from build123d import *

# Parameters (mm, degrees)
SKETCH1_W           = 160
SKETCH1_H           = 180
BOSS_EXTRUDE1_DEPTH = 19.05
SKETCH2_W           = 160
SKETCH2_H           = 180
SKETCH2_W_2         = 147.3
SKETCH2_H_2         = 167.3
BOSS_EXTRUDE2_DEPTH = 44.680000048
SKETCH3_R           = 6.253999938
CUT_EXTRUDE1_DEPTH  = 12.7
SKETCH4_W           = 19.05
SKETCH4_H           = 19.05
SKETCH4_R           = 3.175
BOSS_EXTRUDE3_DEPTH = 12.7


with BuildPart() as part:
    # Sketch1 → Boss-Extrude1 (new body)
    with BuildSketch(Plane(origin=(0, 0, 0), x_dir=(1, 0, 0), z_dir=(0, 1, 0))):
        Rectangle(SKETCH1_W, SKETCH1_H)
    extrude(amount=BOSS_EXTRUDE1_DEPTH)

    # Sketch2 → Boss-Extrude2 (add)
    with BuildSketch(Plane(origin=(0, 19.05, 0), x_dir=(1, 0, 0), z_dir=(0, 1, 0))):
        Rectangle(SKETCH2_W, SKETCH2_H)
        Rectangle(SKETCH2_W_2, SKETCH2_H_2, mode=Mode.SUBTRACT)
    extrude(amount=BOSS_EXTRUDE2_DEPTH)

    # Sketch3 → Cut-Extrude1 (cut)
    with BuildSketch(Plane(origin=(0, 19.05, 0), x_dir=(1, 0, 0), z_dir=(0, 1, 0))):
        with Locations(Location((38.41, -45.55, 0), (0, 0, 270))):
            Circle(SKETCH3_R)
        with Locations(Location((23.17, -45.55, 0), (0, 0, 270))):
            Circle(SKETCH3_R)
        with Locations(Location((38.41, -30.31, 0), (0, 0, 270))):
            Circle(SKETCH3_R)
        with Locations(Location((23.17, -30.31, 0), (0, 0, 270))):
            Circle(SKETCH3_R)
    extrude(amount=-CUT_EXTRUDE1_DEPTH, mode=Mode.SUBTRACT)

    # Sketch4 → Boss-Extrude3 (add)
    # profile 1 of 4: a face of its own
    with BuildSketch(Plane.XZ):
        with Locations((-89.525, -50.08)):
            Rectangle(SKETCH4_W, SKETCH4_H)
        with Locations(Location((-89.525, -50.08, 0), (0, 0, 270))):
            Circle(SKETCH4_R, mode=Mode.SUBTRACT)
    # profile 2 of 4: a face of its own
    with BuildSketch(Plane.XZ):
        with Locations((-89.525, 51.52)):
            Rectangle(SKETCH4_W, SKETCH4_H)
        with Locations(Location((-89.525, 51.52, 0), (0, 0, 270))):
            Circle(SKETCH4_R, mode=Mode.SUBTRACT)
    # profile 3 of 4: a face of its own
    with BuildSketch(Plane.XZ):
        with Locations((89.525, -50.08)):
            Rectangle(SKETCH4_W, SKETCH4_H)
        with Locations(Location((89.525, -50.08, 0), (0, 0, 270))):
            Circle(SKETCH4_R, mode=Mode.SUBTRACT)
    # profile 4 of 4: a face of its own
    with BuildSketch(Plane.XZ):
        with Locations((89.525, 51.52)):
            Rectangle(SKETCH4_W, SKETCH4_H)
        with Locations(Location((89.525, 51.52, 0), (0, 0, 270))):
            Circle(SKETCH4_R, mode=Mode.SUBTRACT)
    extrude(amount=-BOSS_EXTRUDE3_DEPTH)


solid = part.part
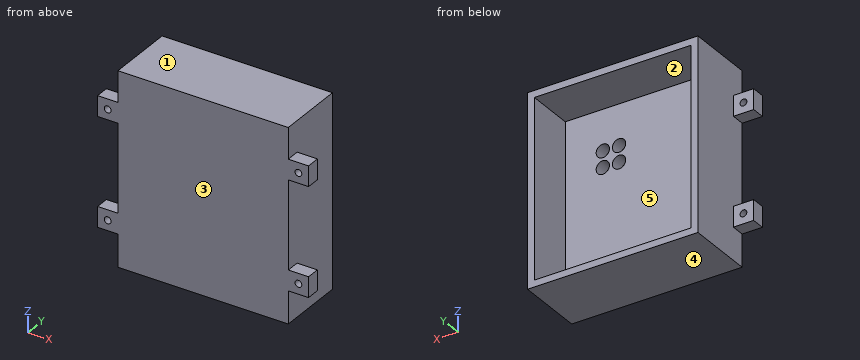
Build history of the part. All positions in model axes, mm. Face numbers are marked on the shaded views. A direction names the side the tool comes from. Round coordinates to 2 decimals unless told otherwise and drop trailing zeros. Write each loop counter-clockwise with the first axis right and the second up, starting at its lowest first coordinate (ties: lowest second). Pieces come first, ordered by that corner, then holes. Notation, with made-up numbers: (38.25, 26.5) - (63.25, 26.5) arc R14 cw to (63.25, 49.5) - close; hole circle Ø9 at (78.25, 5). An arc over 180 degrees is marked (long way). One line per question, with ' | ' between items.
1. Band-saw the part on A-A, the plane z = -50.08. Write the cut outline in (x, y), and give its area (3 significant figures).
Results are:
outline: (-99.05, 0) - (-92.7, 0) - (-92.7, 12.7) - (-99.05, 12.7) - close; (-86.35, 0) - (86.35, 0) - (86.35, 12.7) - (80, 12.7) - (80, 63.73) - (73.65, 63.73) - (73.65, 19.05) - (-73.65, 19.05) - (-73.65, 63.73) - (-80, 63.73) - (-80, 12.7) - (-86.35, 12.7) - close; (92.7, 0) - (99.05, 0) - (99.05, 12.7) - (92.7, 12.7) - close | area: 3,940 mm^2
2. Band-saw the part on D-D, the plane x = -30. Write the cut outline in (y, z), and give its area (3 significant figures).
Results are:
outline: (0, -90) - (63.73, -90) - (63.73, -83.65) - (19.05, -83.65) - (19.05, 83.65) - (63.73, 83.65) - (63.73, 90) - (0, 90) - close | area: 4,000 mm^2
3. Band-saw the part on C-C, the plane z = 45.55. Write the cut outline in (x, y), and give its area (3 significant figures).
Results are:
outline: (-99.05, 0) - (99.05, 0) - (99.05, 12.7) - (80, 12.7) - (80, 63.73) - (73.65, 63.73) - (73.65, 19.05) - (44.66, 19.05) - (44.66, 6.35) - (32.16, 6.35) - (32.16, 19.05) - (29.42, 19.05) - (29.42, 6.35) - (16.92, 6.35) - (16.92, 19.05) - (-73.65, 19.05) - (-73.65, 63.73) - (-80, 63.73) - (-80, 12.7) - (-99.05, 12.7) - close | area: 3,780 mm^2
4. Tool access for the marked faces 4 and 5: list every direction of +Z, -Z, +X, -X, +Y, -Y with a clear straight run to the whole face (end or side of a thin tool).
Results are:
face 4: -Z, +X, -X, +Y, -Y | face 5: +Y
5. Drop flat-ended pins along their axis: pin 1 Ø3 at (y, z) = (33, -32.5) entering from -X; pin 2 Ø1 at (y, z) = (37, 59.5) entering from +X; pin 3 Ø21 at (x, z) = (-86.5, 50.5) entering from +Y; pin 4 Ø2 at (x, z) = (-27.5, -28) entering from +Y. Give the stop position or say it passes through.
Results are:
pin 1: x = -80 | pin 2: x = 80 | pin 3: y = 63.73 | pin 4: y = 19.05
6. Drill centre lines: line 1 along X through (y, z) = (13, 30); line 2 along X through (y, z) = (25.5, 42); line 3 along X through (y, z) = (18, 49.5). Where is each one in solid material? Low to high. Write a range as from..to.
Results are:
line 1: -80..16.92, 29.42..32.16, 44.66..80 | line 2: -80..-73.65, 73.65..80 | line 3: -80..18.32, 28.02..33.56, 43.26..80
7. Mould opens along Z. For the marked faces 1, 2 and 3 say: released by +Z, released by -Z, zero draft, split by the parting line, or undercut.
Results are:
face 1: released by +Z | face 2: undercut | face 3: zero draft
8. Band-saw the part on B-B, the plane y = 45.5. Write the cut outline in (x, z), and give its area (3 significant figures).
Results are:
outline: (-80, -90) - (80, -90) - (80, 90) - (-80, 90) - close; hole (-73.65, -83.65) - (73.65, -83.65) - (73.65, 83.65) - (-73.65, 83.65) - close | area: 4,160 mm^2
